Check sheet for the drawn part. Datum: minimum x, y, z corner. Units: mm. A direction names the side the tool comes from. Give positions to 0.01 mm unless a question says otherwise; leave off trailing zeros. Loops run counter-clockwise (first coordinate to the right, second up) from the corner with the lowest first, then second, coordinate; pieces in that order, holes last.
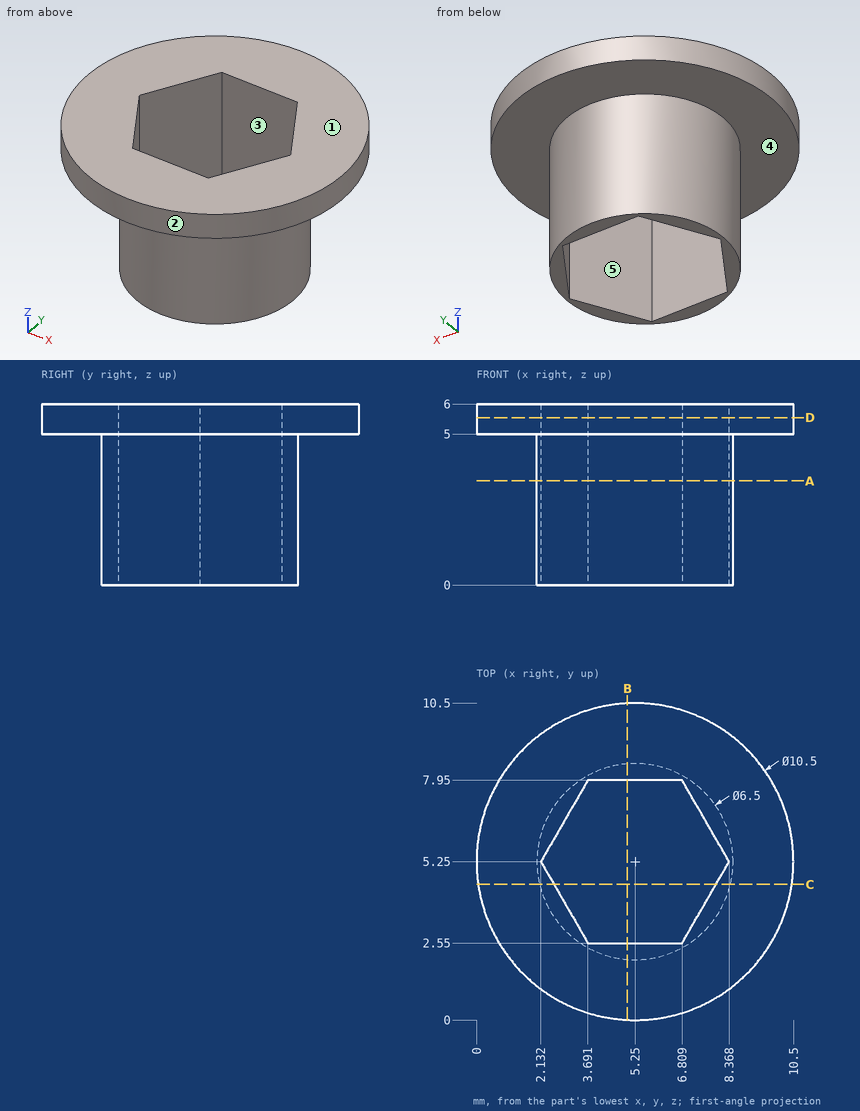
1) Scan lines: line 1 along Y through (x, z) = (5.25, 3.45); line 2 along Z through (x, y) = (9.25, 6); line 3 along X through (y, z) = (6, 4.4) (1 decimal). Record each from-to range of solid material in increasing order.
2) Sectioned sample at D-D on z = 5.55. Enter the section's corners in (x, y).
3) Sectioned sample at C-C on y = 4.5. Enter the section's corners in (x, z) (1 decimal).
4) Depth check by flat-ended pin: P1, Ø2.5, axis at x = 5, z = 2, coming from the -Y side; P2, Ø3, axis at y = 9, z = 2, coming from the -X side (1 decimal); P3, Ø1.5, axis at y = 4, z = 1, coming from the +X side. Enter the tip coordinate at first touch or a pass-through.
5) Tool access check on the marked faces 4 and 5. Record the directions out of +Z, -Z, +X, -X, +Y, -Y that give a thin tool (end or side, any length) a straight path to the whole face; none if there is none.
6) Sectioned sample at B-B on x = 5. Enter the section's corners in (y, z).
7) Sectioned sample at A-A on z = 3.45. Enter the section's corners in (x, y).
8) Mould release check, pull along X, two halves, no side actions. Record for the marked faces 1, 2 and 3: +X half, -X half, draft (parallel to the pull), parting line (faces both ways), or undercut.
Determined:
1. line 1: y = 2 to 2.55, 7.95 to 8.5
1. line 2: z = 5 to 6
1. line 3: x = 2.1 to 2.6, 7.9 to 8.4
2. outline: circle Ø10.5 at (5.25, 5.25); hole (2.13, 5.25) - (3.69, 2.55) - (6.81, 2.55) - (8.37, 5.25) - (6.81, 7.95) - (3.69, 7.95) - close
3. outline: (0.1, 5) - (2.1, 5) - (2.1, 0) - (2.6, 0) - (2.6, 6) - (0.1, 6) - close; (7.9, 0) - (8.4, 0) - (8.4, 5) - (10.4, 5) - (10.4, 6) - (7.9, 6) - close
4. P1: stops at y = 2
4. P2: stops at x = 2.9
4. P3: stops at x = 8.46
5. face 4: -Z
5. face 5: +Z, -Z
6. outline: (0.01, 5) - (2.01, 5) - (2.01, 0) - (2.55, 0) - (2.55, 6) - (0.01, 6) - close; (7.95, 0) - (8.49, 0) - (8.49, 5) - (10.49, 5) - (10.49, 6) - (7.95, 6) - close
7. outline: circle Ø6.5 at (5.25, 5.25); hole (2.13, 5.25) - (3.69, 2.55) - (6.81, 2.55) - (8.37, 5.25) - (6.81, 7.95) - (3.69, 7.95) - close
8. face 1: draft
8. face 2: parting line
8. face 3: undercut
